```python
from build123d import *


with BuildPart() as part:
    # Sketch1 → Revolve1 (revolve)
    with BuildSketch(Plane(origin=(0, 0, 0), x_dir=(0, 0, -1), z_dir=(1, 0, 0))):
        with BuildLine():
            Line((-0.8255, 93.6625), (0.8255, 93.6625))
            ThreePointArc((0.8255, 93.6625), (1.364315367, 93.439315367), (1.5875, 92.9005))
            Line((1.5875, 92.9005), (1.5875, 91.2495))
            ThreePointArc((1.5875, 91.2495), (1.364315367, 90.710684633), (0.8255, 90.4875))
            Line((0.8255, 90.4875), (-0.8255, 90.4875))
            ThreePointArc((-0.8255, 90.4875), (-1.364315367, 90.710684633), (-1.5875, 91.2495))
            Line((-1.5875, 91.2495), (-1.5875, 92.9005))
            ThreePointArc((-1.5875, 92.9005), (-1.364315367, 93.439315367), (-0.8255, 93.6625))
        make_face()
    revolve(axis=Axis((0, 0, 0), (0, 0, 1)))


solid = part.part
```
Part model, mm, in its own coordinate system. Coordinates: 2 decimals unless noted, no trailing zeros. Loops run counter-clockwise (first coordinate to the right, second up) from the corner with the lowest first, then second, coordinate; pieces in that order, holes last. Notation, with made-up numbers: (29, 45.25) - (59, 45.25) arc R32 ccw to (59, 76.25) - close; hole circle Ø4 at (66, 68.25). An arc over 180 degrees is marked (long way). Write item = value, one per line. Start each with the question number.
Item 1: Mould opens along Y. For faces 1 (the flat face through (68, 62, -1.588)), 2 (the cylindrical face through (-89.717, -11.78, 0.012)), 3 (the cylindrical face through (-28.13, 89.34, -0.01)) say: released by +Y, released by -Y, zero draft, split by the parting line, or undercut.
Item 2: Cut at A-A, the plane x = 0. Give the cut face in (y, z), and give its area (3 significant figures).
Item 3: Wall check: L1, parallel to X at y = 0, z = -0.4; L2, parallel to X at y = -61, z = 1.2. Give the ranges that are in metal, low to high. Write a range as from..to.
The answers:
q1.face_1 = zero draft
q1.face_2 = undercut
q1.face_3 = split by the parting line
q2.outline = (-93.66, -0.83) arc R0.76 ccw to (-92.9, -1.59) - (-91.25, -1.59) arc R0.76 ccw to (-90.49, -0.83) - (-90.49, 0.83) arc R0.76 ccw to (-91.25, 1.59) - (-92.9, 1.59) arc R0.76 ccw to (-93.66, 0.83) - close; (90.49, -0.83) arc R0.76 ccw to (91.25, -1.59) - (92.9, -1.59) arc R0.76 ccw to (93.66, -0.83) - (93.66, 0.83) arc R0.76 ccw to (92.9, 1.59) - (91.25, 1.59) arc R0.76 ccw to (90.49, 0.83) - close
q2.area = 19.2 mm2
q3.L1 = -93.66..-90.49, 90.49..93.66
q3.L2 = -70.95..-66.97, 66.97..70.95
